Geometry check sheet. Reference: the model listing, model coordinates, mm. Face numbers are marked on the shaded views. A direction names the side the tool comes from. Round coordinates to 2 decimals unless told otherwise and drop trailing zeros. Write each loop counter-clockwise with the first axis right and the second up, starting at its lowest first coordinate (ties: lowest second). Pieces come first, ordered by that corner, then holes.
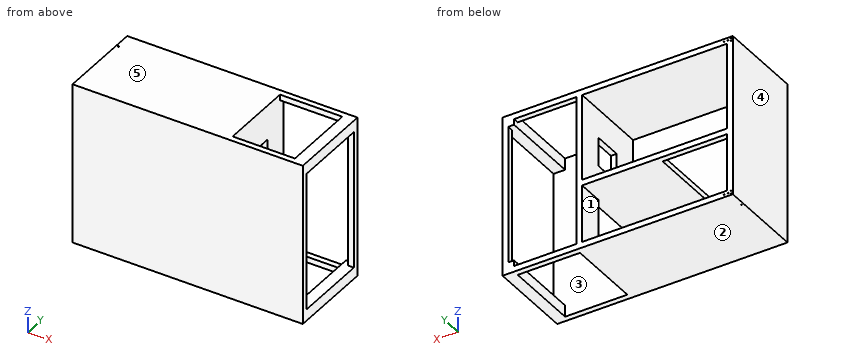
from build123d import *

# Parameters (mm, degrees)
SKETCH1_W               = 2000
SKETCH1_H               = 1400
BOSS_EXTRUDE1_DEPTH     = 50
SKETCH2_W               = 100
SKETCH2_H               = 100
SKETCH2_W_2             = 50
SKETCH2_H_2             = 1300
SKETCH2_W_3             = 718
SKETCH2_H_3             = 50
BOSS_EXTRUDE2_DEPTH     = 700
SKETCH3_W               = 50
SKETCH3_H               = 50
BOSS_EXTRUDE3_DEPTH     = 591
SKETCH4_W               = 50
SKETCH4_H               = 750
BOSS_EXTRUDE4_DEPTH     = 700
SKETCH5_W               = 250
SKETCH5_H               = 250
CUT_EXTRUDE1_DEPTH      = 700
SKETCH6_W               = 50
SKETCH6_H               = 225
BOSS_EXTRUDE5_DEPTH     = 500
SKETCH8_W               = 50
SKETCH8_H               = 50
BOSS_EXTRUDE6_DEPTH     = 541
SKETCH9_W               = 50
SKETCH9_H               = 50
BOSS_EXTRUDE7_DEPTH     = 1200
CUT_EXTRUDE3_DEPTH      = 2554.918557824
CUT_EXTRUDE3_DEPTH_BACK = 2554.918557824
SKETCH11_R              = 5
CUT_EXTRUDE4_DEPTH      = 2554.918557824
CUT_EXTRUDE4_DEPTH_BACK = 10
SKETCH12_R              = 4


with BuildPart() as part:
    # Sketch1 → Boss-Extrude1 (new body)
    with BuildSketch(Plane(origin=(0, 0, 0), x_dir=(1, 0, 0), z_dir=(0, 1, 0))):
        with Locations((1000, 700)):
            Rectangle(SKETCH1_W, SKETCH1_H)
    extrude(amount=BOSS_EXTRUDE1_DEPTH)

    # Sketch2 → Boss-Extrude2 (add)
    with BuildSketch(Plane(origin=(0, 50, 0), x_dir=(1, 0, 0), z_dir=(0, 1, 0))):
        with Locations((1950, 1350)):
            Rectangle(SKETCH2_W, SKETCH2_H)
        with Locations((1950, 50)):
            Rectangle(SKETCH2_W, SKETCH2_H)
        Polygon((0, 1400), (0, 1350), (50, 1350), (1359, 1350), (1359, 1400), align=None)
        with Locations((25, 700)):
            Rectangle(SKETCH2_W_2, SKETCH2_H_2)
        Polygon((50, 50), (0, 50), (0, 0), (1359, 0), (1359, 50), align=None)
        with Locations((1000, 825)):
            Rectangle(SKETCH2_W_3, SKETCH2_H_3)
    extrude(amount=BOSS_EXTRUDE2_DEPTH)

    # Sketch3 → Boss-Extrude3 (add)
    with BuildSketch(Plane.ZY.offset(-641)):
        with Locations((-825, 725)):
            Rectangle(SKETCH3_W, SKETCH3_H)
    extrude(amount=BOSS_EXTRUDE3_DEPTH)

    # Sketch4 → Boss-Extrude4 (add)
    with BuildSketch(Plane(origin=(0, 50, 0), x_dir=(1, 0, 0), z_dir=(0, 1, 0))):
        with Locations((1334, 425)):
            Rectangle(SKETCH4_W, SKETCH4_H)
    extrude(amount=BOSS_EXTRUDE4_DEPTH)

    # Sketch5 → Cut-Extrude1 (cut)
    with BuildSketch(Plane(origin=(1359, 0, 0), x_dir=(0, 0, -1), z_dir=(1, 0, 0))):
        with Locations((425, 400)):
            Rectangle(SKETCH5_W, SKETCH5_H)
    extrude(amount=-CUT_EXTRUDE1_DEPTH, mode=Mode.SUBTRACT)

    # Sketch6 → Boss-Extrude5 (add)
    with BuildSketch(Plane.XY.offset(-1350)):
        with Locations((1334, 637.5)):
            Rectangle(SKETCH6_W, SKETCH6_H)
    extrude(amount=BOSS_EXTRUDE5_DEPTH)

    # Sketch8 → Boss-Extrude6 (add)
    with BuildSketch(Plane(origin=(1359, 0, 0), x_dir=(0, 0, -1), z_dir=(1, 0, 0))):
        with Locations((25, 725)):
            Rectangle(SKETCH8_W, SKETCH8_H)
        with Locations((1375, 725)):
            Rectangle(SKETCH8_W, SKETCH8_H)
    extrude(amount=BOSS_EXTRUDE6_DEPTH)

    # Sketch9 → Boss-Extrude7 (add)
    with BuildSketch(Plane.XY.offset(-1300)):
        with Locations((1975, 725)):
            Rectangle(SKETCH9_W, SKETCH9_H)
    extrude(amount=BOSS_EXTRUDE7_DEPTH)

    # Sketch11 → Cut-Extrude3 (cut, two sides: drawn at the far end of the back side and taken through both)
    with BuildSketch(Plane.XY.offset(-CUT_EXTRUDE3_DEPTH_BACK)):
        with Locations((20, 600)):
            Circle(SKETCH11_R)
    extrude(amount=CUT_EXTRUDE3_DEPTH + CUT_EXTRUDE3_DEPTH_BACK, mode=Mode.SUBTRACT)

    # Sketch12 → Cut-Extrude4 (cut, two sides: drawn at the far end of the back side and taken through both)
    with BuildSketch(Plane(origin=(0, 750, 0), x_dir=(1, 0, 0), z_dir=(0, 1, 0)).offset(-CUT_EXTRUDE4_DEPTH_BACK)):
        with Locations(Location((14.5, 36, 0), (0, 0, 270))):
            Circle(SKETCH12_R)
        with Locations(Location((14.5, 12, 0), (0, 0, 270))):
            Circle(SKETCH12_R)
        with Locations(Location((41.5, 24, 0), (0, 0, 270))):
            Circle(SKETCH12_R)
        with Locations(Location((75.5, 24, 0), (0, 0, 270))):
            Circle(SKETCH12_R)
        with Locations(Location((14.5, 1388, 0), (0, 0, 270))):
            Circle(SKETCH12_R)
        with Locations(Location((14.5, 1364, 0), (0, 0, 270))):
            Circle(SKETCH12_R)
        with Locations(Location((41.5, 1376, 0), (0, 0, 270))):
            Circle(SKETCH12_R)
        with Locations(Location((75.5, 1376, 0), (0, 0, 270))):
            Circle(SKETCH12_R)
    extrude(amount=CUT_EXTRUDE4_DEPTH + CUT_EXTRUDE4_DEPTH_BACK, mode=Mode.SUBTRACT)


solid = part.part
1. Scan lines: line 1 along Z through (x, y) = (789, 271); line 2 along Z through (x, y) = (184, 401); line 3 along X through (y, z) = (600, -726). Record each from-to range of solid material in increasing order.
2. Depth check by flat-ended pin: pin 1 Ø6 at (x, z) = (832.5, -1136) entering from -Y; pin 2 Ø6.5 at (x, z) = (14.5, -12) entering from +Y; pin 3 Ø1 at (y, z) = (295.5, -853) entering from +X. Enter the tip coordinate at first touch or a pass-through.
3. Section check B-B (y = 654.5). Record the cut outline in (x, z), plus the area to 3 significant figures.
4. Release check for a two-part mould opening along Z. For the marked faces 3, 4 and 5 record: +Z half, -Z half, draft (parallel to the pull), parting line (faces both ways), or undercut.
5. Access from +Z, -Z, +X, -X, +Y, -Y to the whole of each face (thin tool, end or side, straight path). Record for the marked faces 1 and 2.
6. Section check D-D (x = 226.5). Record the cut outline in (y, z), plus the area to 4 significant figures.
7. Section check A-A (z = -222.5). Record the cut outline in (x, y), plus the area to 3 significant figures.
8. Section check C-C (y = 110). Record the cut outline in (x, z).
Results below:
1. line 1: z = -1400 to -1350, -850 to -800, -50 to 0
1. line 2: z = -1400 to -1350, -50 to 0
1. line 3: x = 0 to 15, 25 to 50, 1309 to 1359
2. pin 1: stops at y = 0
2. pin 2: stops at y = 740
2. pin 3: stops at x = 50
3. outline: (0, -1400) - (1359, -1400) - (1359, 0) - (0, 0) - close; (1900, -1400) - (2000, -1400) - (2000, -1300) - (1900, -1300) - close; (1900, -100) - (2000, -100) - (2000, 0) - (1900, 0) - close; hole (50, -1350) - (1309, -1350) - (1309, -850) - (641, -850) - (641, -800) - (1309, -800) - (1309, -50) - (50, -50) - close
3. area: 319,000 mm2
4. face 3: undercut
4. face 4: draft
4. face 5: +Z half
5. face 1: +Y
5. face 2: -Z, +X, -X, +Y, -Y
6. outline: (0, -1400) - (750, -1400) - (750, -1350) - (50, -1350) - (50, -50) - (750, -50) - (750, 0) - (0, 0) - close; (700, -850) - (750, -850) - (750, -800) - (700, -800) - close
6. area: 142,500 mm2
7. outline: (0, 0) - (2000, 0) - (2000, 50) - (1359, 50) - (1359, 750) - (1309, 750) - (1309, 50) - (50, 50) - (50, 750) - (0, 750) - close; (1950, 700) - (2000, 700) - (2000, 750) - (1950, 750) - close; hole circle Ø10 at (20, 600)
7. area: 172,000 mm2
8. outline: (0, -1400) - (1359, -1400) - (1359, -1350) - (50, -1350) - (50, -50) - (1309, -50) - (1309, -800) - (641, -800) - (641, -850) - (1359, -850) - (1359, 0) - (0, 0) - close; (1900, -1400) - (2000, -1400) - (2000, -1300) - (1900, -1300) - close; (1900, -100) - (2000, -100) - (2000, 0) - (1900, 0) - close
